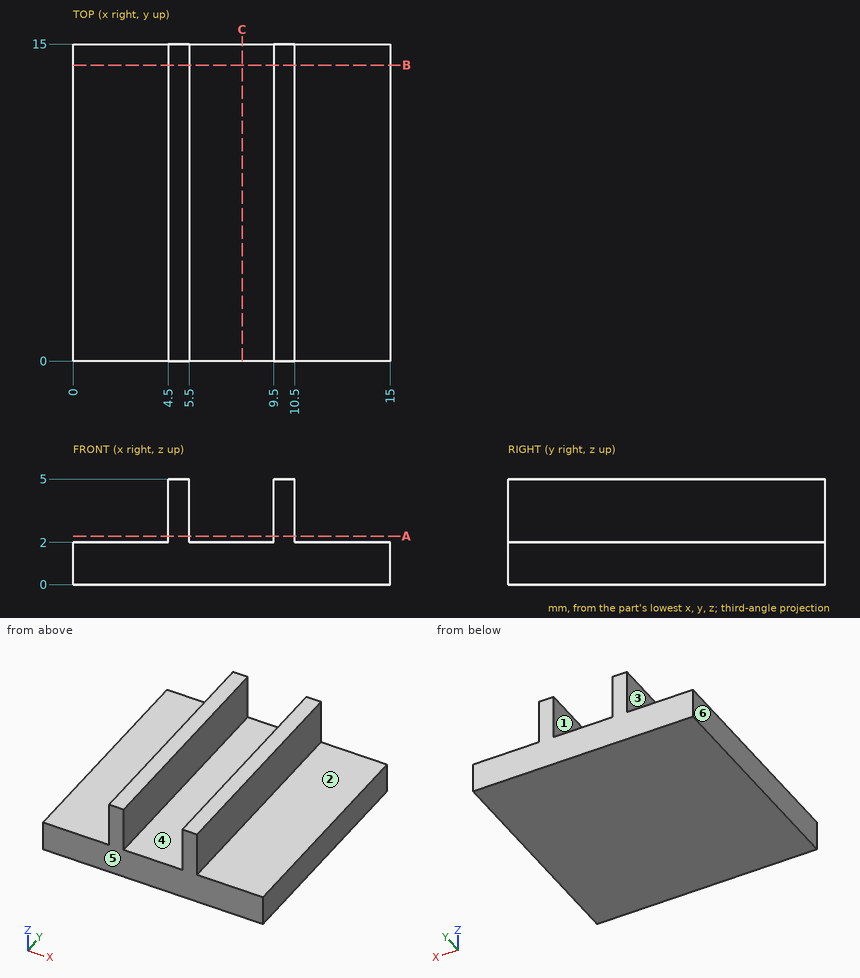
Print and shaded views of the part. All mm, measured from the part's lowest x, y and z. A direction names the side the tool comes from. Give positions to 0.01 mm unless a question says otherwise; leave off trailing zeros. Write each loop counter-clockwise with the first axis right and the second up, starting at its lowest first coordinate (ties: lowest second). Pieces come first, ordered by that corner, then holes. Notation, with made-up numbers: (72, -32.75) - (115, -32.75) arc R25 ccw to (115, -16.75) - close; hole circle Ø1 at (-39, 17.5). An arc over 180 degrees is marked (long way). Put each result on its own line as item: value.
(1) Drop flat-ended pins along their axis: pin 1 Ø1.5 at (y, z) = (4, 4) entering from +X; pin 2 Ø0.9 at (y, z) = (5, 3.5) entering from -X; pin 3 Ø2 at (x, y) = (13.5, 4.5) entering from +Z; pin 4 Ø5 at (x, y) = (3, 6.5) entering from +Z. Give the stop position or say it passes through.
Working result:
pin 1: x = 10.5
pin 2: x = 4.5
pin 3: z = 2
pin 4: z = 5
(2) Saw through at A-A (z = 2.3). List the corners of the cut face in (x, y).
Working result:
outline: (4.5, 0) - (5.5, 0) - (5.5, 15) - (4.5, 15) - close; (9.5, 0) - (10.5, 0) - (10.5, 15) - (9.5, 15) - close
(3) Saw through at B-B (y = 14). List the corners of the cut face in (x, z), then the cut area to 3 significant figures.
Working result:
outline: (0, 0) - (15, 0) - (15, 2) - (10.5, 2) - (10.5, 5) - (9.5, 5) - (9.5, 2) - (5.5, 2) - (5.5, 5) - (4.5, 5) - (4.5, 2) - (0, 2) - close
area: 36.0 mm^2
(4) Pull direction X, two halves, no side cores. Call the marked faces 4, 5 and 6: released by +X, released by -X, zero draft, split by the parting line, or undercut.
Working result:
face 4: undercut
face 5: zero draft
face 6: released by -X
(5) Tool access for the marked faces 1, 2 and 3: list every direction of +Z, -Z, +X, -X, +Y, -Y with a clear straight run to the whole face (end or side of a thin tool).
Working result:
face 1: +Z, +Y, -Y
face 2: +Z, +X, +Y, -Y
face 3: +Z, -X, +Y, -Y
(6) Saw through at C-C (x = 8). List the corners of the cut face in (y, z).
Working result:
outline: (0, 0) - (15, 0) - (15, 2) - (0, 2) - close
(7) Wall check: L1, parallel to X at y = 7.75, z = 3.8; L2, parallel to Z at x = 8.25, y = 4.75. Give the ranges that are in metal, low to high.
Working result:
L1: 4.5 to 5.5, 9.5 to 10.5
L2: 0 to 2
